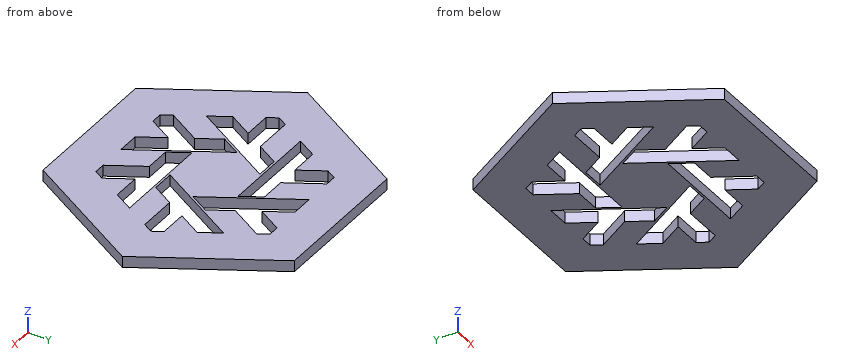
from build123d import *

# Parameters (mm, degrees)
PAD_DEPTH = 10


with BuildPart() as part:
    # Sketch → Pad (new body)
    with BuildSketch(Plane.XY):
        Polygon((130, 0), (65, 112.583302), (-65, 112.583302), (-130, 0), (-65, -112.583302), (65, -112.583302), align=None)
        Polygon((35, 77.942286), (22.5, 56.291651), (10, 77.942286), (-10, 77.942286), (33.845299, 2), (43.845299, 19.320508), (32.5, 38.971143), (50, 69.282032), (45, 77.942286), align=None, mode=Mode.SUBTRACT)
        Polygon((85, -8.660254), (50, -8.660254), (38.654701, -28.310889), (18.654701, -28.310889), (62.5, 47.631397), (72.5, 30.310889), (60, 8.660254), (85, 8.660254), (90, 0), align=None, mode=Mode.SUBTRACT)
        Polygon((35, -77.942286), (17.5, -47.631397), (-5.190599, -47.631397), (-15.190599, -30.310889), (72.5, -30.310889), (62.5, -47.631397), (37.5, -47.631397), (50, -69.282032), (45, -77.942286), align=None, mode=Mode.SUBTRACT)
        Polygon((-85, -8.660254), (-60, -8.660254), (-72.5, -30.310889), (-62.5, -47.631397), (-18.654701, 28.310889), (-38.654701, 28.310889), (-50, 8.660254), (-85, 8.660254), (-90, 0), align=None, mode=Mode.SUBTRACT)
        Polygon((-50, 69.282032), (-45, 77.942286), (-35, 77.942286), (-17.5, 47.631397), (5.190599, 47.631397), (15.190599, 30.310889), (-72.5, 30.310889), (-62.5, 47.631397), (-37.5, 47.631397), align=None, mode=Mode.SUBTRACT)
        Polygon((-35, -77.942286), (-22.5, -56.291651), (-10, -77.942286), (10, -77.942286), (-33.845299, -2), (-43.845299, -19.320508), (-32.5, -38.971143), (-50, -69.282032), (-45, -77.942286), align=None, mode=Mode.SUBTRACT)
    extrude(amount=PAD_DEPTH)


solid = part.part
Read the model definition and answer for the solid it produces. Units are mm, in the model's axes. Coordinates: 2 decimals unless noted, no trailing zeros. Loops run counter-clockwise (first coordinate to the right, second up) from the corner with the lowest first, then second, coordinate; pieces in that order, holes last.
Q1. The part is cut by section B-B on y = -52.5. Write down the section's boundary in (x, z).
Q2. The part is cut by section D-D on z = 2.5. Give the number of separate pieces and of enclosed holes in the cut face, and give its area (3 significant figures).
Q3. The part is cut by section A-A on y = -12.5. Write down the section's boundary in (x, z).
Q4. Consider probe 1 along X at (y, z) = (-70.5, 4.75); probe 2 along Y at (x, z) = (-27.5, 6.25); probe 3 along X at (y, z) = (45, 2.5). Determine where each line is inside the solid, lowest interval first.
Q5. The part is cut by section C-C on x = -69. Write down the section's boundary in (y, z).
Q6. Each of these flat-tipped pins is pushed along its axis until it touches: pin 1 Ø5 at (y, z) = (20, 3.5) entering from -X; pin 2 Ø3 at (x, z) = (-74, 7) entering from -Y; pin 3 Ø1 at (y, z) = (-52, 2.5) entering from -X; pin 4 Ø8 at (x, y) = (49, 13) entering from -Z. Where does it stop, or does it pass through?
Results below:
1. outline: (-99.69, 0) - (-40.31, 0) - (-40.31, 10) - (-99.69, 10) - close; (-4.69, 0) - (20.31, 0) - (20.31, 10) - (-4.69, 10) - close; (40.31, 0) - (99.69, 0) - (99.69, 10) - (40.31, 10) - close
2. separate pieces: 1
2. enclosed holes: 6
2. area: 32,500 mm2
3. outline: (-122.78, 0) - (-62.22, 0) - (-62.22, 10) - (-122.78, 10) - close; (-42.22, 0) - (-39.91, 0) - (-39.91, 10) - (-42.22, 10) - close; (-27.78, 0) - (27.78, 0) - (27.78, 10) - (-27.78, 10) - close; (47.78, 0) - (122.78, 0) - (122.78, 10) - (47.78, 10) - close
4. probe 1: x = -89.3 to -49.3, -30.7 to -14.3, 5.7 to 30.7, 49.3 to 89.3
4. probe 2: y = -112.58 to -64.95, -12.99 to 12.99, 28.31 to 30.31, 64.95 to 112.58
4. probe 3: x = -104.02 to -64.02, 6.71 to 9.02, 35.98 to 60.98, 64.02 to 104.02
5. outline: (-105.66, 0) - (-36.37, 0) - (-36.37, 10) - (-105.66, 10) - close; (-24.25, 0) - (-8.66, 0) - (-8.66, 10) - (-24.25, 10) - close; (8.66, 0) - (30.31, 0) - (30.31, 10) - (8.66, 10) - close; (36.37, 0) - (105.66, 0) - (105.66, 10) - (36.37, 10) - close
6. pin 1: stops at x = -119.9
6. pin 2: stops at y = -99.59
6. pin 3: stops at x = -100.27
6. pin 4: passes through
